Here's how the part is built. I have some questions about the finished solid (model axes, mm). Give positions to 0.01 mm unless a question says otherwise; leave off trailing zeros. Loops run counter-clockwise (first coordinate to the right, second up) from the corner with the lowest first, then second, coordinate; pieces in that order, holes last. Notation, with made-up numbers: M 31.25,42.25 L 84.25,42.25 A18 cw 84.25,46.25 Z; hole C -10.75,60.25 d3. An arc over 180 degrees is marked long. Answer as CSV lines item,"result". Start each with the question number.
Item 1: I want a section at B-B on z = 2.4. List the corners of the cut face in (x, y) for me, plus the area to 3 significant figures.
Item 2: I want a section at C-C on y = 32.5. List the corners of the cut face in (x, z) for me.
Item 3: I want a section at A-A on x = -25. List the corners of the cut face in (y, z) for me, plus the area to 3 significant figures.
Item 4: I want a section at D-D on x = -14. List the corners of the cut face in (y, z) for me, plus the area to 3 significant figures.
Item 5: If I drill on line 1 along Y through (x, z) = (-22.5, 1.4); line 2 along Y through (x, z) = (4.5, 4); line 3 along X through (y, z) = (21, 4.6), over which ranges is the centre line in solid material (lowest first)? Write a range as from..to.
Item 6: Will these pins go through, and if not, where does the flat tip stop? P1, Ø1, axis at y = -12, z = 2.5, coming from the +X side; P2, Ø1, axis at y = 0, z = 4, coming from the -X side; P3, Ø1.5, axis at y = 76, z = 4, coming from the +X side.
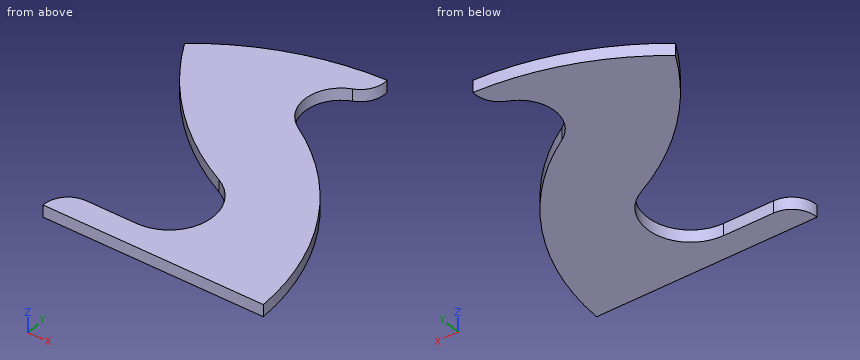
from build123d import *

# Parameters (mm, degrees)
BOSS_EXTRUDE1_DEPTH = 5


with BuildPart() as part:
    # Sketch1 → Boss-Extrude1 (new body)
    with BuildSketch(Plane.XY):
        with BuildLine():
            ThreePointArc((14.997095472, 79.753001356), (19.811312597, 83.805122165), (21.252071738, 89.930526859))
            ThreePointArc((21.252071738, 89.930526859), (-12.511912674, 83.267872862), (-42.835125453, 66.992112713))
            ThreePointArc((-42.835125453, 66.992112713), (-21.592512505, 37.387836987), (7.997709308, 16.125651795))
            ThreePointArc((7.997709308, 16.125651795), (17.525149533, -4.107205113), (0, -18))
            Line((0, -18), (-20.016448778, -18))
            ThreePointArc((-20.016448778, -18), (-27.087516589, -20.928932188), (-30.016448778, -28))
            Line((-30.016448778, -28), (57.983551222, -28))
            ThreePointArc((57.983551222, -28), (45.893125435, 18.420717493), (12.694098189, 53.045650682))
            ThreePointArc((12.694098189, 53.045650682), (5.610650395, 67.109432367), (14.997095472, 79.753001356))
        make_face()
    extrude(amount=BOSS_EXTRUDE1_DEPTH)


solid = part.part
Result:
1,outline,"M -42.84,66.99 A112.5 ccw 8,16.13 A18 cw 0,-18 L -20.02,-18 A10 ccw -30.02,-28 L 57.98,-28 A95.16 ccw 12.69,53.05 A15 cw 15,79.75 A10 ccw 21.25,89.93 A116 ccw Z"
1,area,"5,460 mm^2"
2,outline,"M -16.39,0 L 36.28,0 L 36.28,5 L -16.39,5 Z"
3,outline,"M -28,0 L -19.33,0 L -19.33,5 L -28,5 Z; M 40.95,0 L 77.95,0 L 77.95,5 L 40.95,5 Z"
3,area,"228 mm^2"
4,outline,"M -28,0 L -18,0 L -18,5 L -28,5 Z; M 30.45,0 L 82.72,0 L 82.72,5 L 30.45,5 Z"
4,area,"311 mm^2"
5,line 1,"-28..-18.31, 38.31..79.16"
5,line 2,"-28..-17.43, 17.94..87.93"
5,line 3,"-0.82..44.4"
6,P1,"x = 56.71"
6,P2,"x = 17.99"
6,P3,"x = 10.28"
